The listing builds one solid part. Answer for the finished solid, in the listing's coordinates (mm). Coordinates: 2 decimals unless noted, no trailing zeros. Write each loop counter-clockwise with the first axis right and the second up, starting at its lowest first coordinate (ties: lowest second). Pieces come first, ordered by that corner, then holes.
(1) The part is cut by section C-C on z = 129. Determine the outline of the cut face in (x, y).
(2) The part is cut by section D-D on x = -44. Determine the outline of the cut face in (y, z).
(3) Straight lines are drawn through the part: line 1 (X direction, y = -79, z = 115); line 2 (Z direction, x = -11, y = -102); line 3 (Z direction, x = -183, y = -100). For each, find the intervals that lie inside material, in ascending order.
(4) The part is cut by section A-A on y = -47. Determine the outline of the cut face in (x, z), plus the area to 3 significant figures.
(5) Given P1, Ø2.5, axis at x = 1.5, z = 56.5, coming from the -Y side; P2, Ø1.5, axis at x = -258, z = -1.5, coming from the -Y side; P3, Ø4, axis at y = -15, z = -3, coming from the -X side, each flat-ended and moving along its own axis, determine where each tip first touches the part or whether it passes through.
(6) For a pull along X with two mould halves and no side action, classify faces 1 (the flat face through (-50, 1, -5)), 2 (the flat face through (-150, -2, 0)), 3 (the flat face through (5, -30, 51)) as +X half, -X half, draft (parallel to the pull), parting line (faces both ways), or undercut.
(7) The part is cut by section B-B on x = -214.5. Determine the outline of the cut face in (y, z).
from build123d import *

# Parameters (mm, degrees)
F1_DEPTH = 115
F2_W     = 20
F2_H     = 140
F3_DEPTH = 5
F4_W     = 25
F4_H     = 100
F5_DEPTH = 5


with BuildPart() as f1:
    # F0 (on Front) → F1 (new body, symmetric)
    with BuildSketch(Plane.XZ):
        Polygon((-300, 0), (0, 0), (0, 120), (-300, 160), align=None)
    extrude(amount=F1_DEPTH, both=True)

    # F2 (on Top) → F3 (join)
    with BuildSketch(Plane.XY):
        with Locations((-260, 0)):
            Rectangle(F2_W, F2_H)
        with Locations((-50, 0)):
            Rectangle(F2_W, F2_H)
    extrude(amount=-F3_DEPTH)

    # F4 (on Right) → F5 (join)
    with BuildSketch(Plane.YZ):
        with Locations((30, 50)):
            Rectangle(F4_W, F4_H)
        with Locations((-30, 50)):
            Rectangle(F4_W, F4_H)
    extrude(amount=F5_DEPTH)


solid = f1.part
Model answer:
1. outline: (-300, -115) - (-67.5, -115) - (-67.5, 115) - (-300, 115) - close
2. outline: (-115, 0) - (-70, 0) - (-70, -5) - (70, -5) - (70, 0) - (115, 0) - (115, 125.87) - (-115, 125.87) - close
3. line 1: x = -300 to 0
3. line 2: z = 0 to 121.47
3. line 3: z = 0 to 144.4
4. outline: (-300, 0) - (-270, 0) - (-270, -5) - (-250, -5) - (-250, 0) - (-60, 0) - (-60, -5) - (-40, -5) - (-40, 0) - (0, 0) - (0, 120) - (-300, 160) - close
4. area: 42,200 mm2
5. P1: stops at y = -42.5
5. P2: stops at y = -70
5. P3: stops at x = -270
6. face 1: draft
6. face 2: undercut
6. face 3: +X half
7. outline: (-115, 0) - (115, 0) - (115, 148.6) - (-115, 148.6) - close
